Input: dimensioned drawing with shaded views. Units: mm. Origin: part minimum x, y, z. A direction names the side the tool comes from. Give positions to 0.01 mm unless a question says otherwise; leave off trailing zeros. Loops run counter-clockwise (first coordinate to the right, second up) from the corner with the lowest first, then second, coordinate; pieces in that order, holes last. Notation, with made-up numbers: (48.25, -4) -> (54.25, -4) arc R11 cw to (54.25, 13) -> close; hole circle Ø2 at (-32.5, 57.25). An arc over 180 degrees is marked (long way). Answer in a Markdown table with one row per item. Add a question column.
1) Section query A-A (x = 4.2). Return the cut outline in (y, z), plus the area to 3 significant figures.
2) Access query for the marked faces 1, 2, 3 and 4. Directions: +Z, -Z, +X, -X, +Y, -Y. A direction counts if a zero-diameter tool reaches every point of the face in a straight line with its end or side. Return the directions, or none.
3) Draft query along Z for the marked faces 5, 6 and 7. Return one class per face: +Z half, -Z half, draft (parallel to the pull), parting line (faces both ways), or undercut.
4) Section query D-D (z = 13.5). Return the cut outline in (x, y), plus the area to 4 significant figures.
5) First-contact query: P1, Ø1.4, axis at x = 3, z = 13.5, coming from the -Y side; P2, Ø2, axis at x = 3.5, z = 8.5, coming from the -Y side; P3, Ø2, axis at x = 3, z = 15.5, coming from the +Y side. Flat tips, straight axial feed; report the tip coordinate or a pass-through.
6) Section query B-B (y = 2.5). Return the cut outline in (x, z), plus the area to 3 significant figures.
7) Section query C-C (x = 2). Return the cut outline in (y, z).
8) Line query: line 1 (Z direction, x = 1.15, y = 4); line 2 (Z direction, x = 3.55, y = 4.6); line 3 (Z direction, x = 0.75, y = 0.35). Output: solid intervals per line, ascending. Write a range as from..to.
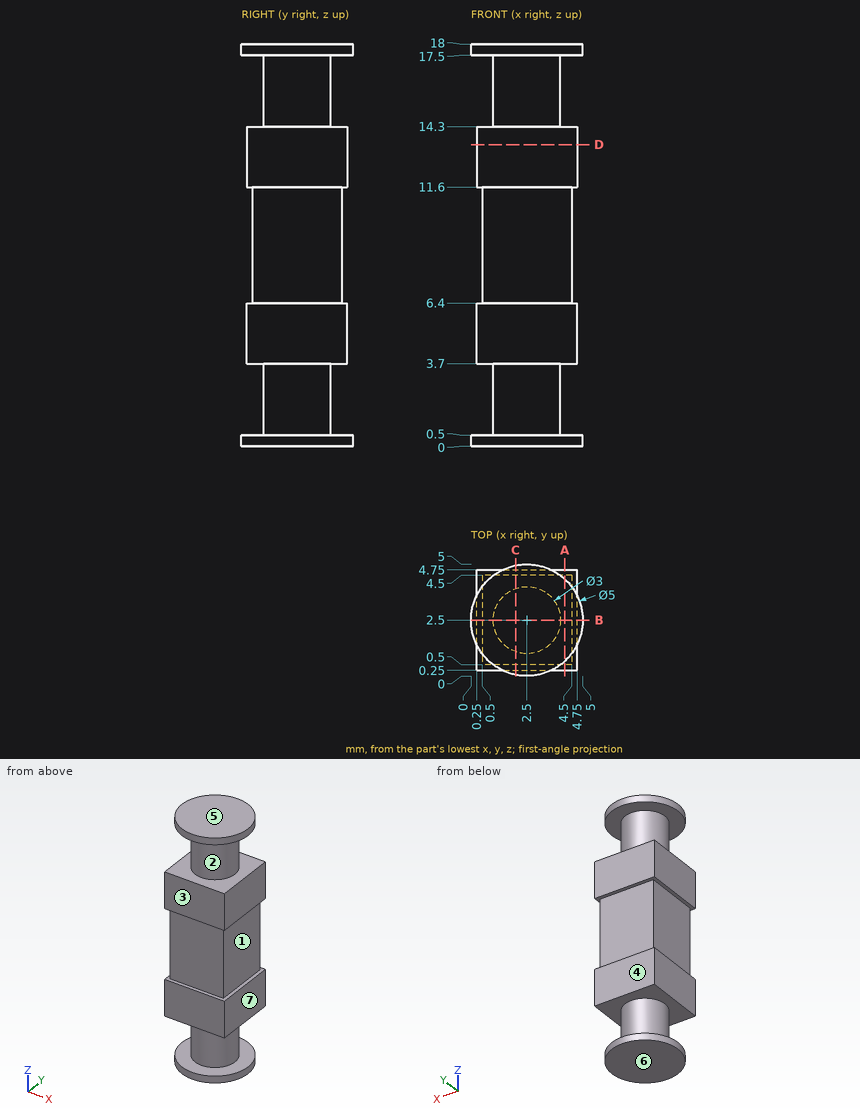
Evaluation:
| question | item | result |
|---|---|---|
| 1 | outline | (0.25, 3.7) -> (4.75, 3.7) -> (4.75, 6.4) -> (4.5, 6.4) -> (4.5, 11.6) -> (4.75, 11.6) -> (4.75, 14.3) -> (0.25, 14.3) -> (0.25, 11.6) -> (0.5, 11.6) -> (0.5, 6.4) -> (0.25, 6.4) -> close; (0.67, 0) -> (4.33, 0) -> (4.33, 0.5) -> (0.67, 0.5) -> close; (0.67, 17.5) -> (4.33, 17.5) -> (4.33, 18) -> (0.67, 18) -> close |
| 1 | area | 48.8 mm² |
| 2 | face 1 | +X, +Y, -Y |
| 2 | face 2 | none |
| 2 | face 3 | +X, -X, -Y |
| 2 | face 4 | +X, -X, +Y |
| 3 | face 5 | +Z half |
| 3 | face 6 | -Z half |
| 3 | face 7 | undercut |
| 4 | outline | (0.25, 0.25) -> (4.75, 0.25) -> (4.75, 4.75) -> (0.25, 4.75) -> close |
| 4 | area | 20.25 mm² |
| 5 | P1 | y = 0.25 |
| 5 | P2 | y = 0.5 |
| 5 | P3 | y = 4 |
| 6 | outline | (0, 0) -> (5, 0) -> (5, 0.5) -> (4, 0.5) -> (4, 3.7) -> (4.75, 3.7) -> (4.75, 6.4) -> (4.5, 6.4) -> (4.5, 11.6) -> (4.75, 11.6) -> (4.75, 14.3) -> (4, 14.3) -> (4, 17.5) -> (5, 17.5) -> (5, 18) -> (0, 18) -> (0, 17.5) -> (1, 17.5) -> (1, 14.3) -> (0.25, 14.3) -> (0.25, 11.6) -> (0.5, 11.6) -> (0.5, 6.4) -> (0.25, 6.4) -> (0.25, 3.7) -> (1, 3.7) -> (1, 0.5) -> (0, 0.5) -> close |
| 6 | area | 69.3 mm² |
| 7 | outline | (0.05, 0) -> (4.95, 0) -> (4.95, 0.5) -> (3.91, 0.5) -> (3.91, 3.7) -> (4.75, 3.7) -> (4.75, 6.4) -> (4.5, 6.4) -> (4.5, 11.6) -> (4.75, 11.6) -> (4.75, 14.3) -> (3.91, 14.3) -> (3.91, 17.5) -> (4.95, 17.5) -> (4.95, 18) -> (0.05, 18) -> (0.05, 17.5) -> (1.09, 17.5) -> (1.09, 14.3) -> (0.25, 14.3) -> (0.25, 11.6) -> (0.5, 11.6) -> (0.5, 6.4) -> (0.25, 6.4) -> (0.25, 3.7) -> (1.09, 3.7) -> (1.09, 0.5) -> (0.05, 0.5) -> close |
| 8 | line 1 | 0..0.5, 3.7..14.3, 17.5..18 |
| 8 | line 2 | 0..0.5, 3.7..6.4, 11.6..14.3, 17.5..18 |
| 8 | line 3 | 3.7..6.4, 11.6..14.3 |
